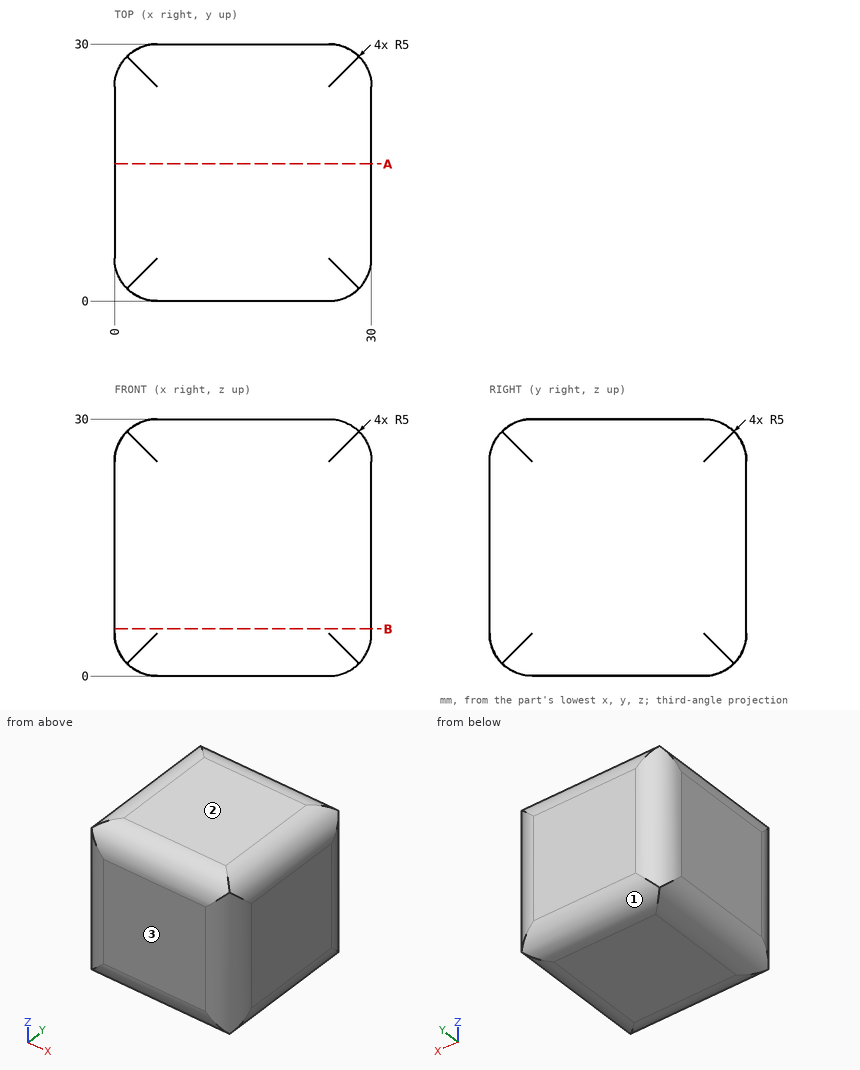
Design review of the part shown in the three views and the two pictorial views. Dimensions are in mm from the part's minimum x, y and z. Give positions to 0.01 mm unless a question says otherwise; leave off trailing zeros. Write each loop counter-clockwise with the first axis right and the second up, starting at its lowest first coordinate (ties: lowest second). Pieces come first, ordered by that corner, then holes.
(1) Mouldability with a two-part tool opening along Z and no side actions: class the marked faces 1, 2 and 3 as +Z half, -Z half, draft (parallel to the pull), parting line (faces both ways), or undercut.
Checked values:
face 1: -Z half
face 2: +Z half
face 3: draft
(2) Clearance check with flat-ended pins moving along their axes: pin 1 Ø3 at (x, y) = (17.5, 3) entering from -Z; pin 2 Ø2 at (y, z) = (14.5, 3) entering from -X. State where each tip first meets the part, or that it passes through.
Checked values:
pin 1: stops at z = 0.03
pin 2: stops at x = 0.1
(3) Wall thickness on line 1 along Y through (x, z) = (28.5, 26); line 2 along Y through (x, z) = (26.5, 15); line 3 along Z through (x, y) = (12, 3): over which ranges is each line inside the solid? List them lowest first.
Checked values:
line 1: y = 1.43 to 28.57
line 2: y = 0.23 to 29.77
line 3: z = 0.42 to 29.58
(4) Add section A-A (y = 16). Give the boundary of the cut face in (x, z).
Checked values:
outline: (0, 5) arc R5 ccw to (5, 0) - (25, 0) arc R5 ccw to (30, 5) - (30, 25) arc R5 ccw to (25, 30) - (5, 30) arc R5 ccw to (0, 25) - close
